Verification items for the finished model (mm, model axes). Give positions to 0.01 mm unless a question says otherwise; leave off trailing zeros. Order: outer loops, then holes, each group sorted by start corner. A loop starts at its lowest first (then second) coordinate and runs counter-clockwise, first axis right, second up. Notation, with made-up numbers: (59.25, -14) - (74.25, -14) arc R15 cw to (74.25, -10) - close; hole circle Ø8 at (59, 40). An arc over 180 degrees is marked (long way). Answer as a JSON object with one key per item and string values. Group by question number.
(1) Depth check by flat-ended pin: pin 1 Ø4 at (x, z) = (-12.7, -889) entering from +Y; pin 2 Ø8 at (x, z) = (-12.7, -1435.1) entering from +Y (3 decimals). Enter the tip coordinate at first touch or a pass-through.
(2) Section check B-B (z = -630.5). Record the boundary of the cut face in (x, y) (3 decimals).
(3) Section check A-A (y = 20.75). Record the boundary of the cut face in (x, z) (3 decimals).
(4) Thickness scan on line 1 (X direction, y = 12.75, z = -288.5) (3 decimals); line 2 (Y direction, x = -18.25, z = -1403) (3 decimals). Record the ranges inside material, lowest first.
```python
from build123d import *

# Parameters (mm, degrees)
LOFT1_START        = -1479.55
LOFT1_DEPTH        = 1479.55
SKETCH3_R          = 2.4257
CUT_EXTRUDE1_DEPTH = 7.62
LPATTERN1_COUNT    = 11
LPATTERN1_PITCH    = 136.525


# Read off the part's stored shape, not the designer's step: Loft1
with BuildPart() as part:
    # Loft1 outline → Loft1 (new body)
    with BuildSketch(Plane.XY.offset(LOFT1_START)):
        Polygon((0, 0), (0, 25.4), (-3.175, 25.4), (-3.175, 3.175), (-22.225, 3.175), (-22.225, 25.4), (-25.4, 25.4), (-25.4, 0), align=None)
    extrude(amount=LOFT1_DEPTH)

    # Sketch3 → Cut-Extrude1 (cut, symmetric)
    with BuildSketch(Plane(origin=(0, 0, 0), x_dir=(1, 0, 0), z_dir=(0, 1, 0))):
        with Locations(Location((-12.7, 69.85, 0), (0, 0, 270))):
            Circle(SKETCH3_R)
    cut_extrude1 = extrude(amount=CUT_EXTRUDE1_DEPTH, both=True, mode=Mode.SUBTRACT)

    # LPattern1: Cut-Extrude1 ×11
    with Locations(*[(0, 0, -i * LPATTERN1_PITCH) for i in range(1, LPATTERN1_COUNT)]):
        add(cut_extrude1, mode=Mode.SUBTRACT)


solid = part.part
```
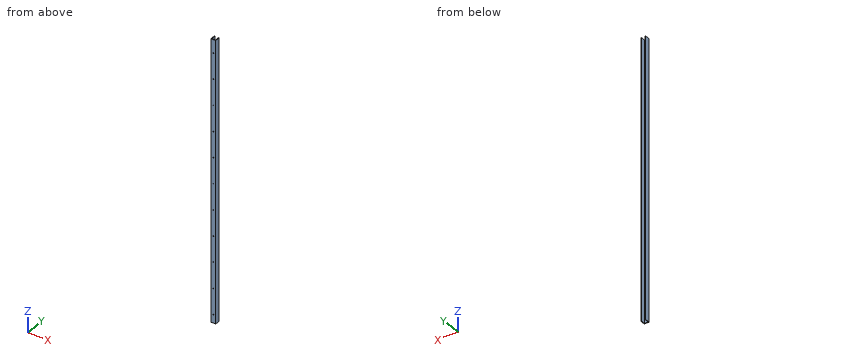
Solutions:
{
 "1": {"pin 1": "passes through", "pin 2": "stops at y = 3.175"},
 "2": {"outline": "(-25.4, 0) - (0, 0) - (0, 25.4) - (-3.175, 25.4) - (-3.175, 3.175) - (-22.225, 3.175) - (-22.225, 25.4) - (-25.4, 25.4) - close"},
 "3": {"outline": "(-25.4, -1479.55) - (-22.225, -1479.55) - (-22.225, 0) - (-25.4, 0) - close; (-3.175, -1479.55) - (0, -1479.55) - (0, 0) - (-3.175, 0) - close"},
 "4": {"line 1": "x = -25.4 to -22.225, -3.175 to 0", "line 2": "y = 0 to 3.175"}
}
